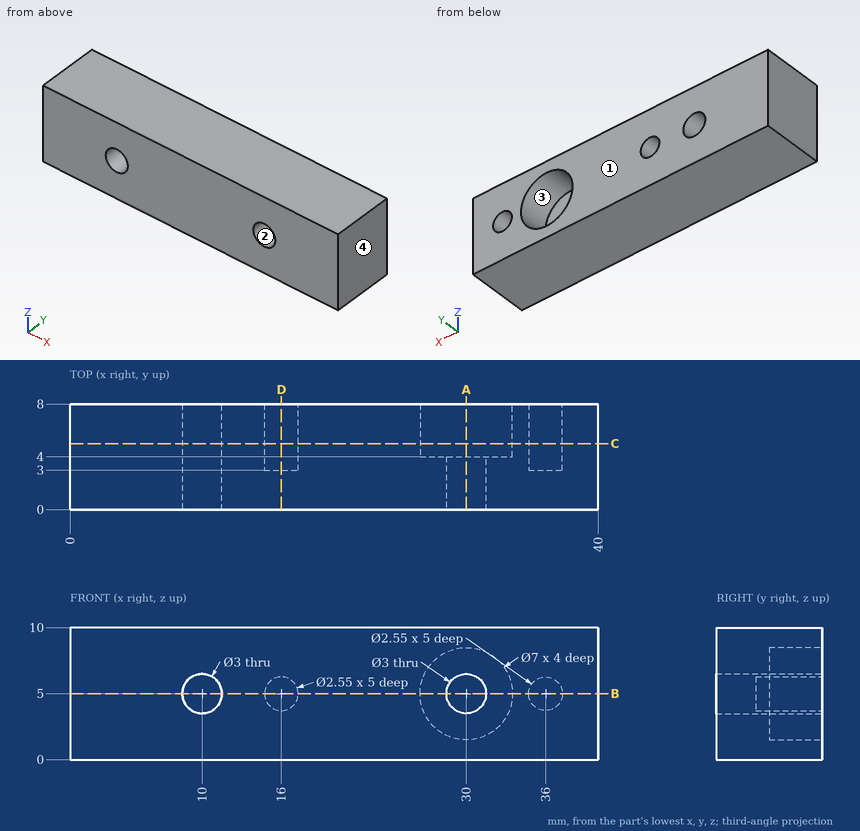
Design review of the part shown in the three views and the two pictorial views. Dimensions are in mm from the part's minimum x, y and z. Round coordinates to 2 decimals unless told otherwise and drop trailing zeros. Loops run counter-clockwise (first coordinate to the right, second up) from the corner with the lowest first, then second, coordinate; pieces in that order, holes last. Notation, with made-up numbers: M 67,36.5 L 91,36.5 A9 cw 91,45.5 Z; hole C -2,75 d10. An arc over 180 degrees is marked long. Answer as a JSON object with one key per item and string values.
Item 1: Wall thickness on L1, parallel to X at y = 5.5, z = 4.25; L2, parallel to X at y = 4.25, z = 4; L3, parallel to Z at x = 30, y = 0.9: over which ranges is each line inside the solid? List them lowest first. Write a range as from..to.
Answer sheet:
{"L1": "x = 0..8.7, 11.3..14.97, 17.03..26.58, 33.42..34.97, 37.03..40", "L2": "x = 0..8.88, 11.12..15.21, 16.79..26.65, 33.35..35.21, 36.79..40", "L3": "z = 0..3.5, 6.5..10"}
Item 2: We need section D-D on x = 16. Give the boundary of the cut face in (y, z) (3 decimals).
Answer sheet:
{"outline": "M 0,0 L 8,0 L 8,3.725 L 3,3.725 L 3,6.275 L 8,6.275 L 8,10 L 0,10 Z"}
Item 3: We need section A-A on x = 30. Give the boundary of the cut face in (y, z), and give its area (3 significant figures).
Answer sheet:
{"outline": "M 0,0 L 8,0 L 8,1.5 L 4,1.5 L 4,3.5 L 0,3.5 Z; M 0,6.5 L 4,6.5 L 4,8.5 L 8,8.5 L 8,10 L 0,10 Z", "area": "40.0 mm^2"}
Item 4: The part is to be moulded in two halves that separate along X. For the marked faces 1, 2, 3 and 4, say which applies: pulls with the +X half, pulls with the -X half, needs draft (parallel to the pull), parting line crosses it, or undercut.
Answer sheet:
{"face 1": "needs draft", "face 2": "undercut", "face 3": "undercut", "face 4": "pulls with the +X half"}
Item 5: Clearance check with flat-ended pins moving along their axes: P1, Ø1.8, axis at x = 30, z = 5, coming from the +Y side; P2, Ø4, axis at x = 30, z = 5, coming from the +Y side. State where each tip first meets the part, or that it passes through.
Answer sheet:
{"P1": "passes through", "P2": "stops at y = 4"}
Item 6: We need section C-C on y = 5. Give the boundary of the cut face in (x, z) (3 decimals), and give its area (3 significant figures).
Answer sheet:
{"outline": "M 0,0 L 40,0 L 40,10 L 0,10 Z; hole C 10,5 d3; hole C 16,5 d2.55; hole C 30,5 d7; hole C 36,5 d2.55", "area": "344 mm^2"}
Item 7: We need section B-B on z = 5. Give the boundary of the cut face in (x, y) (3 decimals).
Answer sheet:
{"outline": "M 0,0 L 8.5,0 L 8.5,8 L 0,8 Z; M 11.5,0 L 28.5,0 L 28.5,4 L 26.5,4 L 26.5,8 L 17.275,8 L 17.275,3 L 14.725,3 L 14.725,8 L 11.5,8 Z; M 31.5,0 L 40,0 L 40,8 L 37.275,8 L 37.275,3 L 34.725,3 L 34.725,8 L 33.5,8 L 33.5,4 L 31.5,4 Z"}
